The listing builds one solid part. Answer for the finished solid, in the listing's coordinates (mm). Face numbers are marked on the shaded views. A direction names the side the tool comes from. Round coordinates to 2 decimals unless told otherwise and drop trailing zeros. Write each loop counter-clockwise with the first axis right and the second up, starting at its lowest first coordinate (ties: lowest second). Pieces come first, ordered by that corner, then holes.
from build123d import *

# Parameters (mm, degrees)
SKETCH_1_W          = 101.7
SKETCH_1_H          = 53.5
EXTRUDE_1_DEPTH     = 1.55
SKETCH_2_R          = 1.7
CUT_EXTRUDE_1_DEPTH = 1.55
SKETCH_3_W          = 16.5
SKETCH_3_H          = 12
EXTRUDE_2_DEPTH     = 10
SKETCH_4_W          = 14
SKETCH_4_H          = 8.7
EXTRUDE_3_DEPTH     = 11
FILLET_1_R          = 4
SKETCH_5_W          = 8.402583841
SKETCH_5_H          = 9.620349616
CUT_EXTRUDE_3_DEPTH = 12.6
SKETCH_6_R          = 3.3
CUT_EXTRUDE_4_DEPTH = 12.6
SKETCH_7_W          = 62.975416122
SKETCH_7_H          = 3.61490304
SKETCH_7_W_2        = 6.088257752
SKETCH_7_H_2        = 41.476255936
SKETCH_7_W_3        = 71.346770532
SKETCH_7_H_3        = 3.044128877
EXTRUDE_4_DEPTH     = 8.5


with BuildPart() as part:
    # 草图1 → 凸台-拉伸1 (new body)
    with BuildSketch(Plane.XY):
        with Locations((1.649757161, 1.28884807)):
            Rectangle(SKETCH_1_W, SKETCH_1_H)
    extrude(amount=EXTRUDE_1_DEPTH)

    # 草图2 → 切除-拉伸1 (cut)
    with BuildSketch(Plane.XY.offset(1.55)):
        with Locations((-34.740242839, -22.86115193)):
            Circle(SKETCH_2_R)
        with Locations((-33.770242839, 25.63884807)):
            Circle(SKETCH_2_R)
        with BuildLine():
            Line((36.418676462, 27.13884807), (47.180837859, 27.13884807))
            ThreePointArc((47.180837859, 27.13884807), (48.880837859, 25.43884807), (47.180837859, 23.73884807))
            Line((47.180837859, 23.73884807), (36.418676462, 23.73884807))
            ThreePointArc((36.418676462, 23.73884807), (34.718676462, 25.43884807), (36.418676462, 27.13884807))
        make_face()
        with BuildLine():
            Line((45.109216811, -21.16115193), (50.49029751, -21.16115193))
            ThreePointArc((50.49029751, -21.16115193), (52.19029751, -22.86115193), (50.49029751, -24.56115193))
            Line((50.49029751, -24.56115193), (45.109216811, -24.56115193))
            ThreePointArc((45.109216811, -24.56115193), (43.409216811, -22.86115193), (45.109216811, -21.16115193))
        make_face()
    extrude(amount=-CUT_EXTRUDE_1_DEPTH, mode=Mode.SUBTRACT)

    # 草图3 → 凸台-拉伸2 (add)
    with BuildSketch(Plane.XY.offset(1.55)):
        with Locations((-47.420242839, 9.956852339)):
            Rectangle(SKETCH_3_W, SKETCH_3_H)
    extrude(amount=EXTRUDE_2_DEPTH)

    # 草图4 → 凸台-拉伸3 (add)
    with BuildSketch(Plane.XY.offset(1.55)):
        with Locations((-45.200242839, -14.884453356)):
            Rectangle(SKETCH_4_W, SKETCH_4_H)
    extrude(amount=EXTRUDE_3_DEPTH)

    # 圆角1
    fillet_1_edges = [part.edges().sort_by_distance(p)[0] for p in [
        (-45.200242839, -10.534453356, 12.55),
        (-45.200242839, -19.234453356, 12.55),
    ]]
    fillet(fillet_1_edges, radius=FILLET_1_R)

    # 草图5 → 切除-拉伸3 (cut)
    with BuildSketch(Plane.ZY.offset(55.670242839)):
        with Locations((6.770558557, 9.995873355)):
            Rectangle(SKETCH_5_W, SKETCH_5_H)
    extrude(amount=-CUT_EXTRUDE_3_DEPTH, mode=Mode.SUBTRACT)

    # 草图6 → 切除-拉伸4 (cut)
    with BuildSketch(Plane.ZY.offset(52.200242839)):
        with Locations((8.55, -14.534453356)):
            Circle(SKETCH_6_R)
    extrude(amount=-CUT_EXTRUDE_4_DEPTH, mode=Mode.SUBTRACT)

    # 草图7 → 凸台-拉伸4 (add)
    with BuildSketch(Plane.XY.offset(1.55)):
        with Locations((0.792982845, 25.166233941)):
            Rectangle(SKETCH_7_W, SKETCH_7_H)
        with Locations((48.072109451, 1.28884807)):
            Rectangle(SKETCH_7_W_2, SKETCH_7_H_2)
        with Locations((4.97866005, -22.30315072)):
            Rectangle(SKETCH_7_W_3, SKETCH_7_H_3)
    extrude(amount=EXTRUDE_4_DEPTH)


solid = part.part
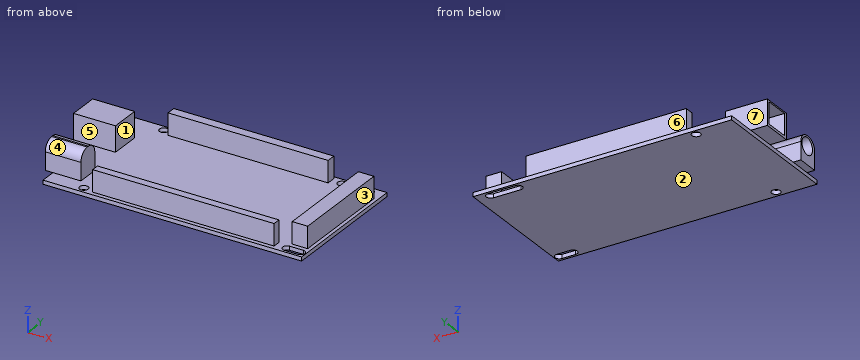
1. Section A-A on x = -46 is taken. Determine the outline of the cut face in (y, z), plus the area to 3 significant figures.
Geometry says:
outline: (-25.46, 0) - (28.04, 0) - (28.04, 1.55) - (15.96, 1.55) - (15.96, 11.55) - (3.96, 11.55) - (3.96, 1.55) - (-10.53, 1.55) - (-10.53, 8.55) arc R4 ccw to (-14.53, 12.55) - (-15.23, 12.55) arc R4 ccw to (-19.23, 8.55) - (-19.23, 1.55) - (-25.46, 1.55) - close; hole circle Ø6.6 at (-14.53, 8.55); hole (5.19, 2.57) - (14.81, 2.57) - (14.81, 10.97) - (5.19, 10.97) - close
area: 177 mm2
2. For a pull along X with two mould halves and no side action, classify the marked faces 1, 2 and 3 as released by +X, released by -X, zero draft, split by the parting line, or undercut.
Geometry says:
face 1: undercut
face 2: zero draft
face 3: released by +X
3. Straight lines are drawn through the part: line 1 along Y through (x, z) = (-46.75, 8.55); line 2 along X through (y, z) = (15.5, 10); line 3 along X through (y, z) = (-13, 4). For each, find the intervals that lie inside material, in ascending order.
Geometry says:
line 1: y = -19.23 to -17.83, -11.23 to -10.53, 3.96 to 5.19, 14.81 to 15.96
line 2: x = -55.67 to -39.17, 45.03 to 51.12
line 3: x = -52.2 to -38.2, 45.03 to 51.12
4. A tool of negligible diameter and unlimited length cuts with its end or side. For the marked faces 4, 5, 6 and 7, from which of +Z, -Z, +X, -X, +Y, -Y can it reach the whole face along a straight path? Write none if from no direction.
Geometry says:
face 4: +Z, -X, -Y
face 5: +Z, -X
face 6: +Z, +X, -X, +Y
face 7: +Z, -X, +Y
5. Section C-C on z = 6.5 is taken. Determine the outline of the cut face in (x, y).
Geometry says:
outline: (-55.67, 3.96) - (-39.17, 3.96) - (-39.17, 15.96) - (-55.67, 15.96) - (-55.67, 14.81) - (-43.07, 14.81) - (-43.07, 5.19) - (-55.67, 5.19) - close; (-52.2, -19.23) - (-38.2, -19.23) - (-38.2, -10.53) - (-52.2, -10.53) - (-52.2, -11.95) - (-39.6, -11.95) - (-39.6, -17.12) - (-52.2, -17.12) - close; (-30.69, -23.83) - (40.65, -23.83) - (40.65, -20.78) - (-30.69, -20.78) - close; (-30.69, 23.36) - (32.28, 23.36) - (32.28, 26.97) - (-30.69, 26.97) - close; (45.03, -19.45) - (51.12, -19.45) - (51.12, 22.03) - (45.03, 22.03) - close
6. Section D-D on x = -10.5 is taken. Determine the outline of the cut face in (y, z).
Geometry says:
outline: (-25.46, 0) - (28.04, 0) - (28.04, 1.55) - (26.97, 1.55) - (26.97, 10.05) - (23.36, 10.05) - (23.36, 1.55) - (-20.78, 1.55) - (-20.78, 10.05) - (-23.83, 10.05) - (-23.83, 1.55) - (-25.46, 1.55) - close
7. Section B-B on y = -6 is taken. Determine the outline of the cut face in (x, z).
Geometry says:
outline: (-49.2, 0) - (52.5, 0) - (52.5, 1.55) - (51.12, 1.55) - (51.12, 10.05) - (45.03, 10.05) - (45.03, 1.55) - (-49.2, 1.55) - close
8. Given pin 1 (1 mm diameter, centred on x = -14, z = 3.5, fed in from +Y); pin 2 (2 mm diameter, centred on x = -34.74, y = -22.86, fed in from -Z); pin 3 (2.5 mm diameter, centred on y = -22, z = 6, fed in from -X); pin 4 (3 mm diameter, centred on x = 47.5, z = 4.5, fed in from -Y), each flat-ended and moving along its own axis, determine where each tip first touches the part or whether it passes through.
Geometry says:
pin 1: stops at y = 26.97
pin 2: passes through
pin 3: stops at x = -30.69
pin 4: stops at y = -19.45
